Input: part model. Units: mm. Frame: model coordinates. A direction names the side the tool comes from. Give positions to 0.01 mm unless a question says otherwise; leave off trailing zeros. Loops run counter-clockwise (first coordinate to the right, second up) from the corner with the lowest first, then second, coordinate; pieces in that order, holes last. Notation, with made-up numbers: (-17.5, 17) - (41.5, 17) arc R25 ccw to (41.5, 40) - close; hole circle Ø4 at (-30.75, -18.75). An arc over 180 degrees is marked (long way). Answer as a JSON object with one key per item and string values.
from build123d import *

# Parameters (mm, degrees)
SKETCH2_R           = 73.3171
SKETCH2_R_2         = 3.302
SKETCH2_R_3         = 4.7625
BOSS_EXTRUDE1_DEPTH = 3.175
CUT_EXTRUDE1_DEPTH  = 6.35


with BuildPart() as part:
    # Sketch2 → Boss-Extrude1 (new, symmetric)
    with BuildSketch(Plane.XY):
        Circle(SKETCH2_R)
        with Locations((-50.8, 0)):
            Circle(SKETCH2_R_2, mode=Mode.SUBTRACT)
        with Locations((50.8, 0)):
            Circle(SKETCH2_R_2, mode=Mode.SUBTRACT)
        with Locations((0, 23.8125)):
            Circle(SKETCH2_R_3, mode=Mode.SUBTRACT)
        with Locations((0, -23.8125)):
            Circle(SKETCH2_R_3, mode=Mode.SUBTRACT)
    extrude(amount=BOSS_EXTRUDE1_DEPTH, both=True)

    # Sketch3 → Cut-Extrude1 (cut)
    with BuildSketch(Plane(origin=(0, 0, -3.175), x_dir=(-1, 0, 0), z_dir=(0, 0, -1))):
        with BuildLine():
            Line((-27.94, -11.43), (-22.86, -11.43))
            ThreePointArc((-22.86, -11.43), (-19.05, -15.24), (-22.86, -19.05))
            Line((-22.86, -19.05), (-27.94, -19.05))
            ThreePointArc((-27.94, -19.05), (-31.75, -15.24), (-27.94, -11.43))
        make_face()
    cut_extrude1 = extrude(amount=-CUT_EXTRUDE1_DEPTH, mode=Mode.SUBTRACT)

    # Mirror1: Cut-Extrude1 across plane
    add(cut_extrude1.mirror(Plane(origin=(0, 0, 0), x_dir=(0, 0, 1), z_dir=(1, 0, 0))), mode=Mode.SUBTRACT)


solid = part.part
Item 1: Access query for faces 1 (the face through (-1, 1, -3.175)), 2 (the face through (-19.05, -15.16, -0.04)). Directions: +Z, -Z, +X, -X, +Y, -Y. A direction counts if a zero-diameter tool reaches every point of the face in a straight line with its end or side. Return the directions, or none.
Geometry check:
{"face 1": "-Z, +X, -X, +Y, -Y", "face 2": "+Z, -Z"}
Item 2: Cut plane C-C (x = 50.8). Return loops of the section in (y, z) (3 decimals).
Geometry check:
{"outline": "(-52.865, -3.175) - (-3.302, -3.175) - (-3.302, 3.175) - (-52.865, 3.175) - close; (3.302, -3.175) - (52.865, -3.175) - (52.865, 3.175) - (3.302, 3.175) - close"}
Item 3: Cut plane D-D (z = 0). Give the number of separate pieces and of enclosed holes in the cut face, then the cut area to 3 significant figures.
Geometry check:
{"separate pieces": "1", "enclosed holes": "6", "area": "16,500 mm2"}
Item 4: Mould query, pull axis X, two halves, no side actions, for faces 3 (the face through (33.831, -65.045, 0.044)), 4 (the face through (25, -19.05, 0)), 5 (the face through (-1, 1, 3.175)), 6 (the face through (-31.75, -15.32, -0.04)). Classes: released by +X, released by -X, zero draft, split by the parting line, or undercut.
Geometry check:
{"face 3": "split by the parting line", "face 4": "undercut", "face 5": "zero draft", "face 6": "undercut"}
Item 5: Contact query for flat-ended pins moving along their axis: P1, Ø5.5, axis at x = -50.8, y = 0, coming from the -Z side; P2, Ø1.5, axis at x = 13.5, z = -1, coming from the -Y side; P3, Ø2.5, axis at x = 25, z = -0.5, coming from the -Y side; P4, Ø1.5, axis at y = -37.5, z = 2, coming from the -X side. Output: stop coordinate, or through.
Geometry check:
{"P1": "passes through", "P2": "stops at y = -72.2", "P3": "stops at y = -69.36", "P4": "stops at x = -63.44"}
Item 6: Cut plane A-A (x = 0). Return loops of the section in (y, z) (3 decimals).
Geometry check:
{"outline": "(-73.317, -3.175) - (-28.575, -3.175) - (-28.575, 3.175) - (-73.317, 3.175) - close; (-19.05, -3.175) - (19.05, -3.175) - (19.05, 3.175) - (-19.05, 3.175) - close; (28.575, -3.175) - (73.317, -3.175) - (73.317, 3.175) - (28.575, 3.175) - close"}
Item 7: Material intervals for line 1 (Y direction, x = 0, z = -2) (3 decimals); line 2 (X direction, y = -1.5, z = 1); line 3 (X direction, y = -12.5, z = 2.5), sorted ascending. Write a range as [from, to].
Geometry check:
{"line 1": "y = [-73.317, -28.575], [-19.05, 19.05], [28.575, 73.317]", "line 2": "x = [-73.3, -53.74], [-47.86, 47.86], [53.74, 73.3]", "line 3": "x = [-72.24, -30.59], [-20.21, 20.21], [30.59, 72.24]"}
Item 8: Cut plane B-B (y = 0). Return loops of the section in (x, z) (3 decimals), then the cut area to 3 significant figures.
Geometry check:
{"outline": "(-73.317, -3.175) - (-54.102, -3.175) - (-54.102, 3.175) - (-73.317, 3.175) - close; (-47.498, -3.175) - (47.498, -3.175) - (47.498, 3.175) - (-47.498, 3.175) - close; (54.102, -3.175) - (73.317, -3.175) - (73.317, 3.175) - (54.102, 3.175) - close", "area": "847 mm2"}
